```python
from build123d import *

# Parameters (mm, degrees)
F0_R     = 127
F1_DEPTH = 12.7
F3_DEPTH = 25.4
F4_COUNT = 25


with BuildPart() as f1:
    # F0 (on Front) → F1 (new body, symmetric)
    with BuildSketch(Plane.XZ):
        Circle(F0_R)
    extrude(amount=F1_DEPTH, both=True)

    # F2 (on face) → F3 (join)
    with BuildSketch(Plane.XZ.offset(12.7)):
        Polygon((-2.263107348, 144.6492542012), (-17.8864400176, 125.7341451774), (13.9443057634, 126.2321525475), align=None)
    extrude(amount=-F3_DEPTH)

    # F4: F1 ×25 about axis
    f4_axis = Axis((0, 0, 0), (0, -1, 0))


with BuildPart() as f1_1:
    add(f1.part)
    for i in range(1, F4_COUNT):
        add(f1.part.rotate(f4_axis, i * 360 / F4_COUNT))


solid = f1_1.part
```
The model under review builds one solid part; all positions refer to its coordinate system, in mm. A direction names the side the tool comes from. Round coordinates to 2 decimals unless told otherwise and drop trailing zeros. Order: outer loops, then holes, each group sorted by start corner. A loop starts at its lowest first (then second) coordinate and runs counter-clockwise, first axis right, second up. Notation, with made-up numbers: (52, -6.75) -> (80, -6.75) arc R18 ccw to (80, 24.25) -> close; hole circle Ø3 at (-8.75, -20.75). An arc over 180 degrees is marked (long way). Use a Markdown table: item, result.
Q1. Clearance check with flat-ended pins moving along their axes: P1, Ø4, axis at x = 40.5, y = -2, coming from the +Z side; P2, Ø1.5, axis at x = 104.5, y = 7, coming from the -Z side; P3, Ø6, axis at x = -24.5, y = 5, coming from the +Z side. State where each tip first meets the part, or that it passes through.
Values:
| item | result |
|---|---|
| P1 | stops at z = 131.39 |
| P2 | stops at z = -90.74 |
| P3 | stops at z = 132.28 |
Q2. We need section A-A on z = 68.5. Write out the cut boundary in (x, y), then the cut area to 3 significant figures.
Values:
| item | result |
|---|---|
| outline | (-121.03, -12.7) -> (117.74, -12.7) -> (117.74, 12.7) -> (-121.03, 12.7) -> close |
| area | 6,060 mm^2 |
Q3. Tool access review of faces 5 (the flat face through (110.62, -0.18, -78.58)), 6 (the flat face through (44.276, -0.178, -128.002)), 7 (the flat face through (-134.031, -0.178, -19.506)): name each direction out of +Z, -Z, +X, -X, +Y, -Y from which nothing blocks a thin tool from reaching the whole face with its end or side.
Values:
| item | result |
|---|---|
| face 5 | +X, +Y, -Y |
| face 6 | -Z, +Y, -Y |
| face 7 | -X, +Y, -Y |
Q4. For line 1 (Z direction, x = 25.5, y = -0.25); line 2 (Z direction, x = 49, y = 1.75); line 3 (X direction, y = 0.25, z = -23), list the stretches that pass through material, from the lowest coordinate up.
Values:
| item | result |
|---|---|
| line 1 | z = -135.13 to 134.64 |
| line 2 | z = -130.41 to 120.43 |
| line 3 | x = -136.75 to 140.95 |
Q5. We need section B-B on x = 103. Write out the cut boundary in (y, z), then the cut area to 3 significant figures.
Values:
| item | result |
|---|---|
| outline | (-12.7, -90.76) -> (12.7, -90.76) -> (12.7, 81.67) -> (-12.7, 81.67) -> close |
| area | 4,380 mm^2 |
Q6. Mouldability with a two-part tool opening along Z and no side actions: class faces 1 (the flat face through (130.53, -0.18, 36.15)), 2 (the flat face through (59.082, -0.178, -122.153)), 3 (the flat face through (-9.97, -0.18, 135.32)), 4 (the flat face through (-1, 12.7, 3)) as +Z half, -Z half, draft (parallel to the pull), parting line (faces both ways), or undercut.
Values:
| item | result |
|---|---|
| face 1 | undercut |
| face 2 | -Z half |
| face 3 | +Z half |
| face 4 | draft |
